Geometry check sheet. Reference: the model listing, model coordinates, mm. Face numbers are marked on the shaded views. A direction names the side the tool comes from. Give positions to 0.01 mm unless a question says otherwise; leave off trailing zeros. Write each loop counter-clockwise with the first axis right and the second up, starting at its lowest first coordinate (ties: lowest second). Pieces come first, ordered by that corner, then holes. Notation, with made-up numbers: (-11, 70) - (13, 70) arc R33 ccw to (13, 100) - close; hole circle Ø2 at (48, 88). An arc over 180 degrees is marked (long way). Write item = value, one per line. Start each with the question number.
(1) Access from +Z, -Z, +X, -X, +Y, -Y to the whole of each face (thin tool, end or side, straight path). Record for the marked faces 1 and 2.
(2) Thickness scan on L1, parallel to Y at x = 95, z = 167.5; L2, parallel to X at y = 76, z = 164.5; L3, parallel to X at y = 105.5, z = 99. Record the ranges inside material, lowest first.
(3) Section check A-A, the plane z = 166.5. Enter the section's corners in (x, y), plus the area to 3 significant figures.
(4) Depth check by flat-ended pin: pin 1 Ø0.8 at (x, y) = (120, 78) entering from +Z; pin 2 Ø3 at (x, z) = (119.5, 86.5) entering from +Y; pin 3 Ø1.5 at (y, z) = (99, 148) entering from +X. Enter the tip coordinate at first touch or a pass-through.
(5) Section check D-D, the plane z = 125. Enter the section's corners in (x, y), plus the area to 3 significant figures.
(6) Section check C-C, the plane y = 69. Enter the section's corners in (x, z).
(7) Draft check along X on the marked faces 3, 4 and 5. Enter one of: pulls with the +X half, pulls with the -X half, needs draft (parallel to the pull), parting line crosses it, or undercut.
(8) Section check B-B, the plane x = 34.5. Enter the section's corners in (y, z), plus the area to 3 significant figures.
```python
from build123d import *

# Parameters (mm, degrees)
BOSS_EXTRUDE1_DEPTH             = 38.1
CUT_EXTRUDE1_DEPTH              = 100.190170884
CUT_EXTRUDE1_DEPTH_BACK         = 100.190170884
BOSS_EXTRUDE2_REACH             = 101.19
BOSS_EXTRUDE2_DIRECTION_2_REACH = 101.19
CUT_EXTRUDE2_DEPTH              = 100.190170884
CUT_EXTRUDE2_DEPTH_BACK         = 100.190170884
SKETCH5_W                       = 149.86
SKETCH5_H                       = 76.2
BOSS_EXTRUDE4_DEPTH             = 19.05


with BuildPart() as part:
    # Sketch1 → Boss-Extrude1 (new body)
    with BuildSketch(Plane(origin=(44.224720049, 74.891650501, 130.282900288), x_dir=(1, 0, 0), z_dir=(0, 1, 0))):
        Polygon((-73.66, -50.8), (-73.66, -19.05), (-76.2, -19.05), (-76.2, 19.05), (-73.66, 19.05), (-73.66, 50.8), (73.66, 50.8), (73.66, 38.1), (76.2, 38.1), (76.2, -38.1), (73.66, -38.1), (73.66, -50.8), align=None)
    extrude(amount=BOSS_EXTRUDE1_DEPTH)

    # Sketch2 → Cut-Extrude1 (cut, two sides: drawn at the far end of the back side and taken through both)
    with BuildSketch(Plane(origin=(44.224720049, 74.891650501, 130.282900288), x_dir=(1, 0, 0), z_dir=(0, 0, 1)).offset(-CUT_EXTRUDE1_DEPTH_BACK)):
        Polygon((-76.2, 12.7), (-57.783825767, 21.287603079), (-55.084357434, 33.987603079), (-44.45, 38.1), (-76.2, 38.1), align=None)
        Polygon((32.670048754, 38.1), (76.2, 7.62), (76.2, 38.1), align=None)
    extrude(amount=CUT_EXTRUDE1_DEPTH + CUT_EXTRUDE1_DEPTH_BACK, mode=Mode.SUBTRACT)

    # Boss-Extrude2: up to this face of the body (flat: up to its plane)
    boss_extrude2_end = Plane(part.part.faces().sort_by_distance((41.857775963, 91.970339861, 181.082900288))[0])
    # Sketch3 → Boss-Extrude2 (add, up to the picked face)
    with BuildSketch(Plane(origin=(44.224720049, 74.891650501, 130.282900288), x_dir=(1, 0, 0), z_dir=(0, 0, 1)), mode=Mode.PRIVATE) as boss_extrude2_sk1:
        Polygon((-76.2, 0), (-76.2, -12.7), (-68.867651581, 0), align=None)
    boss_extrude2_tool1 = split(extrude(boss_extrude2_sk1.sketch, amount=BOSS_EXTRUDE2_REACH, mode=Mode.PRIVATE), bisect_by=boss_extrude2_end, keep=Keep.BOTH, mode=Mode.PRIVATE)
    # Sketch3 → Boss-Extrude2 (add, up to the picked face)
    with BuildSketch(Plane(origin=(44.224720049, 74.891650501, 130.282900288), x_dir=(1, 0, 0), z_dir=(0, 0, 1)), mode=Mode.PRIVATE) as boss_extrude2_sk2:
        Polygon((76.2, 0), (76.2, -12.7), (68.867651581, 0), align=None)
    boss_extrude2_tool2 = split(extrude(boss_extrude2_sk2.sketch, amount=BOSS_EXTRUDE2_REACH, mode=Mode.PRIVATE), bisect_by=boss_extrude2_end, keep=Keep.BOTH, mode=Mode.PRIVATE)
    add(boss_extrude2_tool1.solids().sort_by(Axis((-29.531164, 70.658317, 130.2829), (0, 0, 1)))[0])
    add(boss_extrude2_tool2.solids().sort_by(Axis((117.980604, 70.658317, 130.2829), (0, 0, 1)))[0])

    # Boss-Extrude2 direction 2: up to this face of the body (flat: up to its plane)
    boss_extrude2_direction_2_end = Plane(part.part.faces().sort_by_distance((41.857775963, 91.970339861, 79.482900288))[0])
    # Sketch3 → Boss-Extrude2 direction 2 (add, up to the picked face)
    with BuildSketch(Plane(origin=(44.224720049, 74.891650501, 130.282900288), x_dir=(1, 0, 0), z_dir=(0, 0, 1)), mode=Mode.PRIVATE) as boss_extrude2_direction_2_sk1:
        Polygon((-76.2, 0), (-76.2, -12.7), (-68.867651581, 0), align=None)
    boss_extrude2_direction_2_tool1 = split(extrude(boss_extrude2_direction_2_sk1.sketch, amount=-BOSS_EXTRUDE2_DIRECTION_2_REACH, mode=Mode.PRIVATE), bisect_by=boss_extrude2_direction_2_end, keep=Keep.BOTH, mode=Mode.PRIVATE)
    # Sketch3 → Boss-Extrude2 direction 2 (add, up to the picked face)
    with BuildSketch(Plane(origin=(44.224720049, 74.891650501, 130.282900288), x_dir=(1, 0, 0), z_dir=(0, 0, 1)), mode=Mode.PRIVATE) as boss_extrude2_direction_2_sk2:
        Polygon((76.2, 0), (76.2, -12.7), (68.867651581, 0), align=None)
    boss_extrude2_direction_2_tool2 = split(extrude(boss_extrude2_direction_2_sk2.sketch, amount=-BOSS_EXTRUDE2_DIRECTION_2_REACH, mode=Mode.PRIVATE), bisect_by=boss_extrude2_direction_2_end, keep=Keep.BOTH, mode=Mode.PRIVATE)
    add(boss_extrude2_direction_2_tool1.solids().sort_by(Axis((-29.531164, 70.658317, 130.2829), (0, 0, -1)))[0])
    add(boss_extrude2_direction_2_tool2.solids().sort_by(Axis((117.980604, 70.658317, 130.2829), (0, 0, -1)))[0])

    # Sketch4 → Cut-Extrude2 (cut, two sides: drawn at the far end of the back side and taken through both)
    with BuildSketch(Plane(origin=(44.224720049, 74.891650501, 130.282900288), x_dir=(0, 0, -1), z_dir=(1, 0, 0)).offset(-CUT_EXTRUDE2_DEPTH_BACK)):
        Polygon((-38.1, 38.1), (-50.8, 25.4), (-50.8, 38.1), align=None)
        Polygon((38.1, 38.1), (50.8, 25.4), (50.8, 38.1), align=None)
    extrude(amount=CUT_EXTRUDE2_DEPTH + CUT_EXTRUDE2_DEPTH_BACK, mode=Mode.SUBTRACT)

    # Sketch5 → Boss-Extrude4 (add)
    with BuildSketch(Plane.XZ.offset(-74.891650501)):
        with Locations((45.494720049, 130.282900288)):
            Rectangle(SKETCH5_W, SKETCH5_H)
    extrude(amount=BOSS_EXTRUDE4_DEPTH)


solid = part.part
```
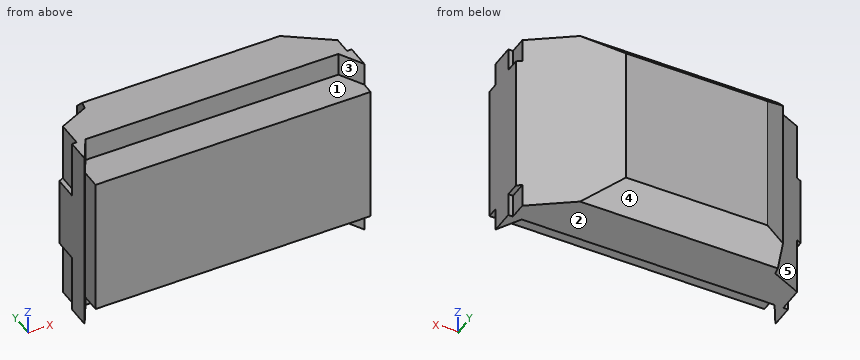
Model answer:
q1.face_1 = +Z, -Y
q1.face_2 = -Z, +X, -X, +Y, -Y
q2.L1 = 55.84 to 100.31
q2.L2 = -29.44 to 120.42
q2.L3 = -11.58 to 87.59
q3.outline = (-31.98, 62.19) - (-29.44, 66.59) - (-29.44, 55.84) - (120.42, 55.84) - (120.42, 82.51) - (76.89, 112.99) - (-0.23, 112.99) - (-10.86, 108.88) - (-13.56, 96.18) - (-29.44, 88.78) - (-29.44, 74.89) - (-31.98, 74.89) - close
q3.area = 7,550 mm²
q4.pin_1 = 168.38
q4.pin_2 = 74.89
q4.pin_3 = 97.95
q5.outline = (-31.98, 62.19) - (-29.44, 66.59) - (-29.44, 55.84) - (120.42, 55.84) - (120.42, 82.51) - (76.89, 112.99) - (-0.23, 112.99) - (-10.86, 108.88) - (-13.56, 96.18) - (-31.98, 87.59) - close
q5.area = 7,590 mm²
q6.outline = (-31.98, 79.48) - (-28.04, 79.48) - (-28.04, 92.18) - (116.49, 92.18) - (116.49, 79.48) - (120.42, 79.48) - (120.42, 181.08) - (116.49, 181.08) - (116.49, 168.38) - (-28.04, 168.38) - (-28.04, 181.08) - (-31.98, 181.08) - close
q7.face_3 = undercut
q7.face_4 = needs draft
q7.face_5 = pulls with the -X half
q8.outline = (55.84, 92.18) - (74.89, 92.18) - (74.89, 79.48) - (100.29, 79.48) - (112.99, 92.18) - (112.99, 168.38) - (100.29, 181.08) - (74.89, 181.08) - (74.89, 168.38) - (55.84, 168.38) - close
q8.area = 5,160 mm²
